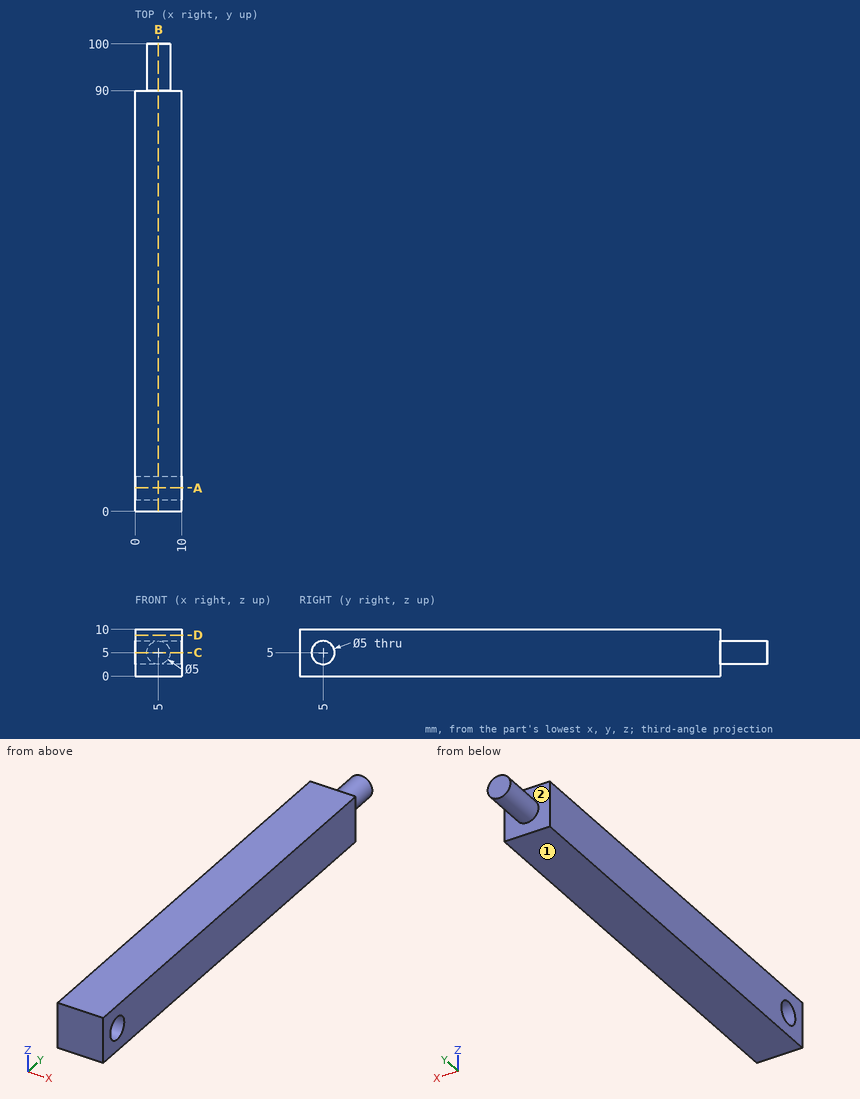
Part print with two shaded views. Sizes in mm from the minimum x, y, z corner. A direction names the side the tool comes from. Coordinates: 2 decimals unless noted, no trailing zeros. Write each loop counter-clockwise with the first axis right and the second up, starting at its lowest first coordinate (ties: lowest second). Pieces come first, ordered by that corner, then holes. Notation, with made-up numbers: (1.25, -40) - (57.25, -40) arc R32 ccw to (57.25, -3) - close; hole circle Ø6 at (47.5, -24.75). An arc over 180 degrees is marked (long way). One line per item, written item: value. Start each with the question number.
1. Probe line 1 (Y direction, x = 2.25, z = 5); line 2 (Y direction, x = 6.75, z = 5); line 3 (Y direction, x = 7.5, z = 9.25). List the from-to ranges inside material, lowest first. Write a range as from..to.
2. Slice it at B-B (x = 5). Write the cut outline in (y, z).
3. Flat gauge pins, fed straight in: pin 1 (2 mm diameter, centred on y = 35, z = 2.5, fed in from -X); pin 2 (3 mm diameter, centred on y = 5, z = 5, fed in from +X). Where does each tip first touch, or does it go through?
4. Tool access for the marked faces 1 and 2: list every direction of +Z, -Z, +X, -X, +Y, -Y with a clear straight run to the whole face (end or side of a thin tool).
5. Slice it at C-C (z = 5). Write the cut outline in (x, y).
6. Slice it at A-A (y = 5). Write the cut outline in (x, z).
7. Slice it at D-D (z = 8.75). Write the cut outline in (x, y), plus the area to 3 significant figures.
Answers below:
1. line 1: y = 0..2.5, 7.5..90
1. line 2: y = 0..2.5, 7.5..100
1. line 3: y = 0..90
2. outline: (0, 0) - (90, 0) - (90, 2.5) - (100, 2.5) - (100, 7.5) - (90, 7.5) - (90, 10) - (0, 10) - close; hole circle Ø5 at (5, 5)
3. pin 1: stops at x = 0
3. pin 2: passes through
4. face 1: -Z, +X, -X, +Y, -Y
4. face 2: +Y
5. outline: (0, 0) - (10, 0) - (10, 2.5) - (0, 2.5) - close; (0, 7.5) - (10, 7.5) - (10, 90) - (7.5, 90) - (7.5, 100) - (2.5, 100) - (2.5, 90) - (0, 90) - close
6. outline: (0, 0) - (10, 0) - (10, 2.5) - (0, 2.5) - close; (0, 7.5) - (10, 7.5) - (10, 10) - (0, 10) - close
7. outline: (0, 0) - (10, 0) - (10, 90) - (0, 90) - close
7. area: 900 mm^2
